Build history of the part. All positions in model axes, mm. A direction names the side the tool comes from. Coordinates: 2 decimals unless noted, no trailing zeros. Write each loop counter-clockwise with the first axis right and the second up, starting at its lowest first coordinate (ties: lowest second). Pieces come first, ordered by that corner, then holes.
```python
from build123d import *

# Parameters (mm, degrees)
SKETCH1_W                = 101.6
SKETCH1_H                = 101.6
SKETCH1_W_2              = 95.25
SKETCH1_H_2              = 95.25
BOSS_EXTRUDE1_DEPTH      = 53.975
CUT_EXTRUDE2_START       = -50.8
CUT_EXTRUDE2_OUTLINE_R   = 5.5626
CUT_EXTRUDE2_OUTLINE_R_2 = 1.905
CUT_EXTRUDE2_DEPTH       = 3.175


# Read off the part's stored shape, not the designer's step: Cut-Extrude2
with BuildPart() as part:
    # Sketch1 → Boss-Extrude1 (new body)
    with BuildSketch(Plane(origin=(0, 0, 0), x_dir=(1, 0, 0), z_dir=(0, 1, 0))):
        Rectangle(SKETCH1_W, SKETCH1_H)
        Rectangle(SKETCH1_W_2, SKETCH1_H_2, mode=Mode.SUBTRACT)
    extrude(amount=BOSS_EXTRUDE1_DEPTH)

    # Cut-Extrude2 outline → Cut-Extrude2 (cut)
    with BuildSketch(Plane.XY.offset(CUT_EXTRUDE2_START)):
        with Locations((-2.5146, 26.289)):
            Circle(CUT_EXTRUDE2_OUTLINE_R)
        with Locations((23.5204, 24.257)):
            Circle(CUT_EXTRUDE2_OUTLINE_R_2)
        with Locations((11.9634, 11.43)):
            Circle(CUT_EXTRUDE2_OUTLINE_R)
        with Locations((-17.4498, 11.43)):
            Circle(CUT_EXTRUDE2_OUTLINE_R)
        with Locations((-17.4498, 24.257)):
            Circle(CUT_EXTRUDE2_OUTLINE_R_2)
    extrude(amount=CUT_EXTRUDE2_DEPTH, mode=Mode.SUBTRACT)


solid = part.part
```
1. Probe line 1 along Z through (x, y) = (-41.5, 3) (3 decimals); line 2 along Z through (x, y) = (0, 24) (3 decimals). List the from-to ranges inside material, lowest first.
Computed values:
line 1: z = -50.8 to -47.625, 47.625 to 50.8
line 2: z = 47.625 to 50.8
2. Saw through at A-A on z = -21. List the corners of the cut face in (x, y) (3 decimals).
Computed values:
outline: (-50.8, 0) - (-47.625, 0) - (-47.625, 53.975) - (-50.8, 53.975) - close; (47.625, 0) - (50.8, 0) - (50.8, 53.975) - (47.625, 53.975) - close
3. Mould opens along Y. For faces 4 (the face through (-4, 0, 49)), 5 (the face through (-19.353, 24.341, -49.235)), 6 (the face through (0.052, 21.354, -49.235)), 7 (the face through (-1, 27, 50.8)) say: +Y half, -Y half, draft (parallel to the pull), parting line (faces both ways), or undercut.
Computed values:
face 4: -Y half
face 5: undercut
face 6: undercut
face 7: draft
4. Saw through at D-D on y = 38. List the corners of the cut face in (x, z) (3 decimals).
Computed values:
outline: (-50.8, -50.8) - (50.8, -50.8) - (50.8, 50.8) - (-50.8, 50.8) - close; hole (-47.625, -47.625) - (47.625, -47.625) - (47.625, 47.625) - (-47.625, 47.625) - close
5. 3-axis set-ups, long thin cutter, end or side, ignore diameter. For faces 1 (the face through (-1, 33, -50.8)), 2 (the face through (21.617, 24.341, -49.235)), 3 (the face through (-1, 33, -47.625)): which of +Z, -Z, +X, -X, +Y, -Y reach the whole face in a straight line?
Computed values:
face 1: -Z, +X, -X, +Y, -Y
face 2: -Z
face 3: +Y, -Y
6. Saw through at B-B on y = 11.43. List the corners of the cut face in (x, z) (3 decimals).
Computed values:
outline: (-50.8, -50.8) - (-23.012, -50.8) - (-23.012, -47.625) - (-47.625, -47.625) - (-47.625, 47.625) - (47.625, 47.625) - (47.625, -47.625) - (17.526, -47.625) - (17.526, -50.8) - (50.8, -50.8) - (50.8, 50.8) - (-50.8, 50.8) - close; (-11.887, -50.8) - (6.401, -50.8) - (6.401, -47.625) - (-11.887, -47.625) - close
7. Flat gauge pin, fed straight in: pin 1 (3.5 mm diameter, centred on x = 23.52, y = 24.26, fed in from -Z) (3 decimals). Where does the tip first touch, or does it go through?
Computed values:
pin 1: stops at z = 47.625
8. Saw through at C-C on x = 5. List the corners of the cut face in (y, z) (3 decimals), plus the area to 3 significant figures.
Computed values:
outline: (0, -50.8) - (53.975, -50.8) - (53.975, -47.625) - (0, -47.625) - close; (0, 47.625) - (53.975, 47.625) - (53.975, 50.8) - (0, 50.8) - close
area: 343 mm2
